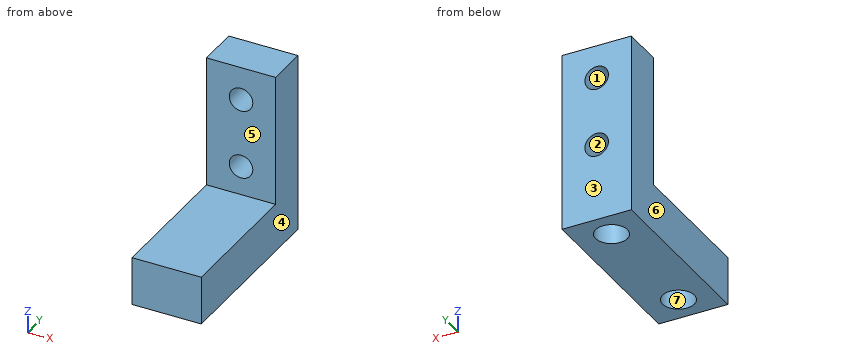
```python
from build123d import *

# Parameters (mm, degrees)
PAD038_DEPTH    = 10
SKETCH109_R     = 2.3
POCKET034_DEPTH = 5.5
SKETCH110_R     = 1.7
HOLE021_DEPTH   = 25


with BuildPart() as part:
    # Sketch108 → Pad038 (new body)
    with BuildSketch(Plane.YZ):
        Polygon((106, 198.8), (106, 205.8), (126, 205.8), (126, 224.8), (132, 224.8), (132, 198.8), align=None)
    extrude(amount=PAD038_DEPTH)

    # Sketch109 (on Face6 of Pad038) → Pocket034 (cut)
    with BuildSketch(Plane.YX.offset(-198.8)):
        with Locations((128, 5)):
            Circle(SKETCH109_R)
        with Locations((110, 5)):
            Circle(SKETCH109_R)
    extrude(amount=-POCKET034_DEPTH, mode=Mode.SUBTRACT)

    # Sketch110 (on Face9 of Pocket034) → Hole021 (cut)
    with BuildSketch(Plane(origin=(0, 126, 0), x_dir=(0, 0, -1), z_dir=(0, -1, 0))):
        with Locations((-220, 5)):
            Circle(SKETCH110_R)
        with Locations((-210, 5)):
            Circle(SKETCH110_R)
    extrude(amount=-HOLE021_DEPTH, mode=Mode.SUBTRACT)


with BuildPart() as part_1:
    # Body015 placement: moved
    add(part.part.moved(Location((-39, 0, 0))))


solid = part_1.part
```
Part model, mm, in its own coordinate system. Face numbers are marked on the shaded views. A direction names the side the tool comes from. Coordinates: 2 decimals unless noted, no trailing zeros. Write each loop counter-clockwise with the first axis right and the second up, starting at its lowest first coordinate (ties: lowest second). Pieces come first, ordered by that corner, then holes.
Item 1: Probe line 1 (Z direction, x = -33.5, y = 126.5); line 2 (X direction, y = 128, z = 202.45); line 3 (X direction, y = 128, z = 210). List the from-to ranges inside material, lowest first.
Item 2: Mould opens along X. For the marked faces 1, 2, 3 and 4 say: released by +X, released by -X, zero draft, split by the parting line, or undercut.
Item 3: Slice it at C-C (x = -34.75). Write the cut outline in (y, z).
Item 4: Pin check, flat tips, straight feed: pin 1 (2 mm diameter, centred on x = -31.5, y = 121, fed in from +Z); pin 2 (5.5 mm diameter, centred on x = -34, z = 220, fed in from +Y); pin 3 (4.5 mm diameter, centred on x = -34, z = 210, fed in from -Y); pin 4 (1.4 mm diameter, centred on x = -33, y = 110, fed in from -Z). Stop position of each tip, or through.
Item 5: Slice it at A-A (z = 220). Write the cut outline in (x, y).
Item 6: Which spindle directions (+Z, -Z, +X, -X, +Y, -Y) get a long thin tool onto all of the face, cutting with end or side? Do the marked faces 5, 6 and 7. Say none if no direction does.
Item 7: Slice it at B-B (y = 128). Write the cut outline in (x, z).
Item 8: Slice it at D-D (z = 201). Write the cut outline in (x, y), and give its area (3 significant figures).
Results found:
1. line 1: z = 204.3 to 208.38, 211.62 to 218.38, 221.62 to 224.8
1. line 2: x = -39 to -36.3, -31.7 to -29
1. line 3: x = -39 to -35.7, -32.3 to -29
2. face 1: undercut
2. face 2: undercut
2. face 3: zero draft
2. face 4: released by +X
3. outline: (106, 198.8) - (107.83, 198.8) - (107.83, 204.3) - (112.17, 204.3) - (112.17, 198.8) - (125.83, 198.8) - (125.83, 204.3) - (130.17, 204.3) - (130.17, 198.8) - (132, 198.8) - (132, 208.47) - (126, 208.47) - (126, 205.8) - (106, 205.8) - close; (126, 211.53) - (132, 211.53) - (132, 218.47) - (126, 218.47) - close; (126, 221.53) - (132, 221.53) - (132, 224.8) - (126, 224.8) - close
4. pin 1: stops at z = 205.8
4. pin 2: stops at y = 132
4. pin 3: stops at y = 126
4. pin 4: stops at z = 204.3
5. outline: (-39, 126) - (-35.7, 126) - (-35.7, 132) - (-39, 132) - close; (-32.3, 126) - (-29, 126) - (-29, 132) - (-32.3, 132) - close
6. face 5: +Z, +X, -X, -Y
6. face 6: +Z, -Z, -X, +Y, -Y
6. face 7: -Z
7. outline: (-39, 198.8) - (-36.3, 198.8) - (-36.3, 204.3) - (-31.7, 204.3) - (-31.7, 198.8) - (-29, 198.8) - (-29, 224.8) - (-39, 224.8) - close; hole circle Ø3.4 at (-34, 210); hole circle Ø3.4 at (-34, 220)
8. outline: (-39, 106) - (-29, 106) - (-29, 132) - (-39, 132) - close; hole circle Ø4.6 at (-34, 110); hole circle Ø4.6 at (-34, 128)
8. area: 227 mm2
